CAD build for the part. Positions are in the model's coordinates, mm. A direction names the side the tool comes from. Coordinates: 2 decimals unless noted, no trailing zeros. Order: outer loops, then holes, each group sorted by start corner. A loop starts at its lowest first (then second) coordinate and runs counter-clockwise, first axis right, second up. Notation, with made-up numbers: (47, 53) - (77, 53) arc R13 cw to (77, 69) - close; hole circle Ø8 at (42, 59). An arc over 180 degrees is marked (long way). Return JSON: item names as keys, results as strings.
from build123d import *

# Parameters (mm, degrees)
SKETCH1_R           = 1.5
BOSS_EXTRUDE1_DEPTH = 10
BOSS_EXTRUDE2_START = -30
BOSS_EXTRUDE2_DEPTH = 30
SKETCH3_W           = 75
SKETCH3_H           = 8
CUT_EXTRUDE1_DEPTH  = 45
CUT_EXTRUDE2_DEPTH  = 7
SKETCH5_R           = 4.5
CUT_EXTRUDE3_DEPTH  = 10
CUT_EXTRUDE4_DEPTH  = 7


with BuildPart() as part:
    # Sketch1 → Boss-Extrude1 (new body)
    with BuildSketch(Plane(origin=(0, 0, 0), x_dir=(1, 0, 0), z_dir=(0, 1, 0))):
        with BuildLine():
            Line((-100, 32.5), (100, 32.5))
            ThreePointArc((100, 32.5), (132.5, 0), (100, -32.5))
            Line((100, -32.5), (-100, -32.5))
            ThreePointArc((-100, -32.5), (-132.5, 0), (-100, 32.5))
        make_face()
        with Locations(Location((85, 15, 0), (0, 0, 270))):
            Circle(SKETCH1_R, mode=Mode.SUBTRACT)
        with Locations(Location((115, 15, 0), (0, 0, 90))):
            Circle(SKETCH1_R, mode=Mode.SUBTRACT)
        with Locations(Location((85, -15, 0), (0, 0, 90))):
            Circle(SKETCH1_R, mode=Mode.SUBTRACT)
        with Locations(Location((115, -15, 0), (0, 0, 270))):
            Circle(SKETCH1_R, mode=Mode.SUBTRACT)
        Polygon((0, 21.5), (-40, 21.5), (-40, 12), (0, 12), (50, 12), (50, 21.5), align=None, mode=Mode.SUBTRACT)
        Polygon((-50, 4.75), (0, 4.75), (65, 4.75), (65, -4.75), (0, -4.75), (-50, -4.75), align=None, mode=Mode.SUBTRACT)
        Polygon((0, -12), (-40, -12), (-40, -21.5), (0, -21.5), (50, -21.5), (50, -12), align=None, mode=Mode.SUBTRACT)
    extrude(amount=BOSS_EXTRUDE1_DEPTH)

    # Sketch2 → Boss-Extrude2 (add)
    with BuildSketch(Plane(origin=(0, 0, 0), x_dir=(1, 0, 0), z_dir=(0, 1, 0)).offset(BOSS_EXTRUDE2_START)):
        with BuildLine():
            Line((-100, 32.5), (100, 32.5))
            ThreePointArc((100, 32.5), (132.5, 0), (100, -32.5))
            Line((100, -32.5), (-100, -32.5))
            ThreePointArc((-100, -32.5), (-132.5, 0), (-100, 32.5))
        make_face()
        with BuildLine():
            Line((99.668543355, 27.510998447), (-100, 27.510998447))
            ThreePointArc((-100, 27.510998447), (-127.55585262, -0.044854173), (-100, -27.600706793))
            Line((-100, -27.600706793), (100.998461852, -27.600706793))
            ThreePointArc((100.998461852, -27.600706793), (128.562336478, 0.636345006), (99.668543355, 27.510998447))
        make_face(mode=Mode.SUBTRACT)
    extrude(amount=BOSS_EXTRUDE2_DEPTH)

    # Sketch3 → Cut-Extrude1 (cut, symmetric)
    with BuildSketch(Plane.XY):
        with Locations((-57.5, -19)):
            Rectangle(SKETCH3_W, SKETCH3_H)
        with Locations((57.5, -19)):
            Rectangle(SKETCH3_W, SKETCH3_H)
        with Locations((57.5, -4)):
            Rectangle(SKETCH3_W, SKETCH3_H)
        with Locations((-57.5, -4)):
            Rectangle(SKETCH3_W, SKETCH3_H)
    extrude(amount=CUT_EXTRUDE1_DEPTH, both=True, mode=Mode.SUBTRACT)

    # Sketch4 → Cut-Extrude2 (cut)
    with BuildSketch(Plane(origin=(0, 0, 0), x_dir=(1, 0, 0), z_dir=(0, 1, 0))):
        Polygon((-102, 19), (-98, 19), (-95.5, 4.5), (-81, 2), (-81, -2), (-95.5, -4.5), (-98, -19), (-102, -19), (-104.5, -4.5), (-119, -2), (-119, 2), (-104.5, 4.5), align=None)
    extrude(amount=CUT_EXTRUDE2_DEPTH, mode=Mode.SUBTRACT)

    # Sketch5 → Cut-Extrude3 (cut)
    with BuildSketch(Plane(origin=(0, 0, 0), x_dir=(1, 0, 0), z_dir=(0, 1, 0))):
        with Locations(Location((-100, 0, 0), (0, 0, 90))):
            Circle(SKETCH5_R)
    extrude(amount=CUT_EXTRUDE3_DEPTH, mode=Mode.SUBTRACT)

    # Sketch7 → Cut-Extrude4 (cut)
    with BuildSketch(Plane.XZ):
        Polygon((-106.5, 4.155172414), (-106.5, -4.155172414), (-104.155172414, -6.5), (-95.844827586, -6.5), (-93.5, -4.155172414), (-93.5, 4.155172414), (-95.844827586, 6.5), (-104.155172414, 6.5), align=None)
    extrude(amount=-CUT_EXTRUDE4_DEPTH, mode=Mode.SUBTRACT)


solid = part.part
Item 1: Drop flat-ended pins along their axis: P1, Ø5, axis at y = -21, z = -14, coming from the -X side; P2, Ø5.5, axis at y = -19.5, z = 30, coming from the -X side; P3, Ø5, axis at x = -26.5, z = -23.5, coming from the -Y side. Give the stop position or say it passes through.
Findings below:
{"P1": "stops at x = -130.4", "P2": "stops at x = -117.71", "P3": "stops at y = 0"}
Item 2: Mould opens along Y. For faces 1 (the flat face through (-1, 0, 8)), 2 (the flat face through (-1, -10, -32.5)), 3 (the flat face through (2, 10, -8)) say: released by +Y, released by -Y, zero draft, split by the parting line, or undercut.
Findings below:
{"face 1": "undercut", "face 2": "zero draft", "face 3": "released by +Y"}
Item 3: Which spindle directions (+Z, -Z, +X, -X, +Y, -Y) get a long thin tool onto all of the face, cutting with end or side? Do faces 4 (the flat face through (1, -19, -27.511)), 5 (the flat face through (20, -4, -30)), 6 (the flat face through (-40, 5, -17)). Say none if no direction does.
Findings below:
{"face 4": "-Y", "face 5": "+Z, -Z", "face 6": "+Y, -Y"}
Item 4: Band-saw the part on A-A, the plane x = -58.5. List the corners of the cut face in (y, z), then the cut area to 3 significant figures.
Findings below:
{"outline": "(-30, -32.5) - (-23, -32.5) - (-23, -27.51) - (-30, -27.51) - close; (-30, 27.6) - (-23, 27.6) - (-23, 32.5) - (-30, 32.5) - close; (-15, -32.5) - (-8, -32.5) - (-8, -27.51) - (-15, -27.51) - close; (-15, 27.6) - (-8, 27.6) - (-8, 32.5) - (-15, 32.5) - close; (0, -32.5) - (10, -32.5) - (10, 32.5) - (0, 32.5) - close", "area": "788 mm²"}
Item 5: Wall check: L1, parallel to Z at x = -5, y = 2; L2, parallel to X at y = 8.5, z = -3; L3, parallel to X at y = 9.15, z = 0. Give the ranges that are in metal, low to high. Write a range as [from, to].
Findings below:
{"L1": "z = [-32.5, -21.5], [-12, -4.75], [4.75, 12], [21.5, 32.5]", "L2": "x = [-132.36, -103.35], [-96.65, -50], [65, 132.36]", "L3": "x = [-132.5, -104.5], [-95.5, -50], [65, 132.5]"}
